```python
from build123d import *


with BuildPart() as part:
    # Sketch1 → Revolve1 (revolve)
    with BuildSketch(Plane(origin=(0, 0, 0), x_dir=(0, 0, -1), z_dir=(1, 0, 0)), mode=Mode.PRIVATE) as revolve1_sk:
        with BuildLine():
            Line((0, -4.5), (-0.95, -4.5))
            ThreePointArc((-0.95, -4.5), (-1.657106781, -4.207106781), (-1.95, -3.5))
            Line((-1.95, -3.5), (-1.95, 2.181346652))
            Line((-1.95, 2.181346652), (-3, 4))
            Line((-3, 4), (-3, 4.5))
            ThreePointArc((-3, 4.5), (-2.707106781, 5.207106781), (-2, 5.5))
            Line((-2, 5.5), (0, 5.5))
            Line((0, 5.5), (0, -4.5))
        make_face()
    revolve(revolve1_sk.sketch.rotate(Axis((0, 0, 0), (0, 1, 0)), 180), axis=Axis((0, 0, 0), (0, 1, 0)))


solid = part.part
```
Input: part model. Units: mm. Frame: model coordinates. A direction names the side the tool comes from. Give positions to 0.01 mm unless a question says otherwise; leave off trailing zeros. Order: outer loops, then holes, each group sorted by start corner. A loop starts at its lowest first (then second) coordinate and runs counter-clockwise, first axis right, second up. Notation, with made-up numbers: M 83.5,29 L 99.5,29 A30 cw 99.5,59 Z; hole C -20,66.5 d8. An arc over 180 degrees is marked long. One line per question, with ' | ' between items. Start each with the question number.
1. Section query A-A (y = -1). Return the cut outline in (x, z).
2. Section query B-B (y = 2.75). Return the cut outline in (x, z).
3. First-contact query: pin 1 Ø1 at (x, y) = (-1, 2.5) entering from -Z; pin 2 Ø1.5 at (y, z) = (-0.5, 1.5) entering from +X; pin 3 Ø3 at (y, z) = (-1, 0) entering from -X. Flat tips, straight axial feed; report the tip coordinate or a pass-through.
4. Material intervals for probe 1 along Z at (x, y) = (-0.1, -3.25); probe 2 along Y at (x, z) = (0.25, -1.4), sorted ascending. Write a range as [from, to].
5. Access query for faces 1 (the face through (0, 5.5, 0)), 2 (the face through (-1.318, -0.62, 1.437)). Directions: +Z, -Z, +X, -X, +Y, -Y. A direction counts if a zero-diameter tool reaches every point of the face in a straight line with its end or side. Return the directions, or none.
Here are the results:
1) outline: C 0,0 d3.9
2) outline: C 0,0 d4.56
3) pin 1: z = -2.26 | pin 2: x = 1.8 | pin 3: x = -1.95
4) probe 1: [-1.95, 1.95] | probe 2: [-4.38, 5.5]
5) face 1: +Z, -Z, +X, -X, +Y | face 2: -Y
